Source: CAD feature listing. Evaluate the final solid. Frame: model axes, mm. Face numbers are marked on the shaded views. A direction names the side the tool comes from. Give positions to 0.01 mm unless a question says otherwise; leave off trailing zeros. Loops run counter-clockwise (first coordinate to the right, second up) from the corner with the lowest first, then second, coordinate; pieces in that order, holes last. Notation, with made-up numbers: (22, 80) -> (63, 80) arc R9 ccw to (63, 89) -> close; hole circle Ø4 at (-24, 26). An arc over 180 degrees is marked (long way). Put each result on its own line as item: value.
```python
from build123d import *

# Parameters (mm, degrees)
ESQUISSE1_W                                        = 30
ESQUISSE1_H                                        = 26
BOSS_EXTRU_1_DEPTH                                 = 60
BOSS_EXTRU_2_DEPTH                                 = 4.5
ESQUISSE3_W                                        = 20.4
ESQUISSE3_H                                        = 20.4
ENL_V_MAT_EXTRU_1_DEPTH                            = 60
D_GAGEMENT_M31_D                                   = 3.4
NERVURE3_REACH                                     = 69.089
ESQUISSE7_WALL_W                                   = 158.445223638
ESQUISSE7_WALL_H                                   = 9
CHAMBRAGE_POUR_VIS_T_TE_HEXAGONALE_M41_D           = 4.5
CHAMBRAGE_POUR_VIS_T_TE_HEXAGONALE_M41_DEPTH       = 4.8
CHAMBRAGE_POUR_VIS_T_TE_HEXAGONALE_M41_CBORE_D     = 8
CHAMBRAGE_POUR_VIS_T_TE_HEXAGONALE_M41_CBORE_DEPTH = 1


with BuildPart() as part:
    # Esquisse1 → Boss.-Extru.1 (new body)
    with BuildSketch(Plane(origin=(0, 0, 0), x_dir=(0, 0, -1), z_dir=(1, 0, 0))):
        with Locations((0, 13)):
            Rectangle(ESQUISSE1_W, ESQUISSE1_H)
    extrude(amount=BOSS_EXTRU_1_DEPTH)

    # Esquisse4 → Boss.-Extru.2 (add, symmetric)
    with BuildSketch(Plane.XY):
        with BuildLine():
            Line((17.5, 0), (17.5, -13.5))
            ThreePointArc((17.5, -13.5), (30, -26), (42.5, -13.5))
            Line((42.5, -13.5), (42.5, 0))
            Line((42.5, 0), (17.5, 0))
        make_face()
    extrude(amount=BOSS_EXTRU_2_DEPTH, both=True)

    # Esquisse3 → Enlèv. mat.-Extru.1 (cut)
    with BuildSketch(Plane.ZY):
        with Locations((0, 13)):
            Rectangle(ESQUISSE3_W, ESQUISSE3_H)
    extrude(amount=-ENL_V_MAT_EXTRU_1_DEPTH, mode=Mode.SUBTRACT)

    # Dégagement M31 (through all)
    with Locations(Plane.XY.offset(4.5)):
        with Locations((30, -13.5)):
            Hole(D_GAGEMENT_M31_D / 2)

    # Esquisse7 wall → Nervure3 (add, up to next)
    with BuildSketch(Plane(origin=(8.75, -6.883592551, 0), x_dir=(0.785943249757, -0.618298639947, 0), z_dir=(0.618298639947, 0.785943249757, 0)), mode=Mode.PRIVATE) as nervure3_sk1:
        Rectangle(ESQUISSE7_WALL_W, ESQUISSE7_WALL_H)
    nervure3_tool1 = extrude(nervure3_sk1.sketch, amount=NERVURE3_REACH, mode=Mode.PRIVATE) - part.part
    add(nervure3_tool1.solids().sort_by_distance((8.75, -6.883592551, 0))[0])

    # Chambrage pour vis à tête hexagonale M41
    with Locations(Plane.XY.offset(15)):
        with Locations((30, 13)):
            chambrage_pour_vis_t_te_hexagonale_m41 = CounterBoreHole(CHAMBRAGE_POUR_VIS_T_TE_HEXAGONALE_M41_D / 2, CHAMBRAGE_POUR_VIS_T_TE_HEXAGONALE_M41_CBORE_D / 2, CHAMBRAGE_POUR_VIS_T_TE_HEXAGONALE_M41_CBORE_DEPTH, depth=CHAMBRAGE_POUR_VIS_T_TE_HEXAGONALE_M41_DEPTH)

    # Symétrie1: Chambrage pour vis à tête hexagonale M41 across plane
    add(chambrage_pour_vis_t_te_hexagonale_m41.mirror(Plane.XY), mode=Mode.SUBTRACT)


solid = part.part
```
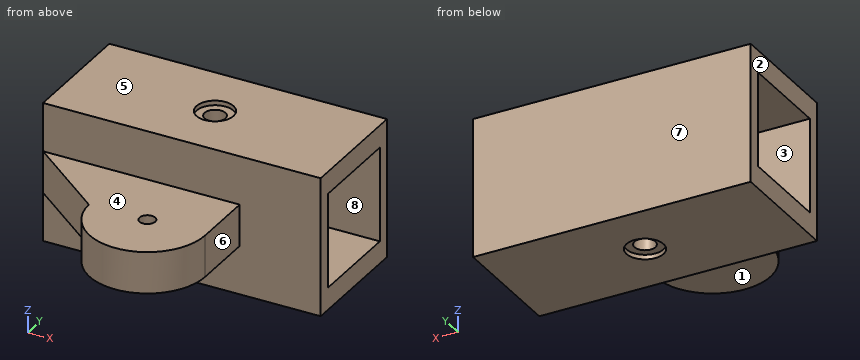
(1) Section B-B on x = 30. Give the number of separate pieces and of enclosed holes in the cut face, then the cut area to 3 significant figures.
Calculated:
separate pieces: 3
enclosed holes: 0
area: 517 mm²
(2) Draft query along Z for the marked faces 1, 2 and 3. Return one class per face: released by +Z, released by -Z, zero draft, split by the parting line, or undercut.
Calculated:
face 1: released by -Z
face 2: zero draft
face 3: undercut
(3) Reachability of the marked faces 4, 5, 6, 7 and 8 from +Z, -Z, +X, -X, +Y, -Y: full face, straight path, thin tool, end or side. Return the list, or none.
Calculated:
face 4: +Z, +X, -X, -Y
face 5: +Z, +X, -X, +Y, -Y
face 6: +Z, -Z, +X, -Y
face 7: +Z, -Z, +X, -X, +Y
face 8: +X, -X
(4) Line query: probe 1 along Y at (x, z) = (30, 1.5); probe 2 along Z at (x, y) = (16, 11); probe 3 along Y at (x, z) = (30, 11.45). Output: solid intervals per line, ascending. Write a range as from..to.
Calculated:
probe 1: y = -26..-15.2, -11.8..2.8, 23.2..26
probe 2: z = -15..-10.2, 10.2..15
probe 3: y = 0..10.75, 15.25..26
(5) Section A-A on z = 2.5. Return loops of the section in (x, y).
Calculated:
outline: (0, 0) -> (17.5, -13.77) arc R12.5 ccw to (42.5, -13.5) -> (42.5, 0) -> (60, 0) -> (60, 2.8) -> (0, 2.8) -> close; (0, 23.2) -> (60, 23.2) -> (60, 26) -> (0, 26) -> close; hole circle Ø3.4 at (30, -13.5)
(6) Section D-D on z = 8.5. Return loops of the section in (x, y).
Calculated:
outline: (0, 0) -> (60, 0) -> (60, 2.8) -> (0, 2.8) -> close; (0, 23.2) -> (60, 23.2) -> (60, 26) -> (0, 26) -> close
(7) Section C-C on y = 18.5. Return loops of the section in (x, z).
Calculated:
outline: (0, -15) -> (60, -15) -> (60, -10.2) -> (0, -10.2) -> close; (0, 10.2) -> (60, 10.2) -> (60, 15) -> (0, 15) -> close
(8) First-contact query: P1, Ø6, axis at x = 30, y = 13, coming from the +Z side; P2, Ø13, axis at x = 20, y = -16.5, coming from the +Z side; P3, Ø4.5, axis at y = -5, z = -1, coming from the +X side. Flat tips, straight axial feed; report the tip coordinate or a pass-through.
Calculated:
P1: stops at z = 14
P2: stops at z = 4.5
P3: stops at x = 42.5
